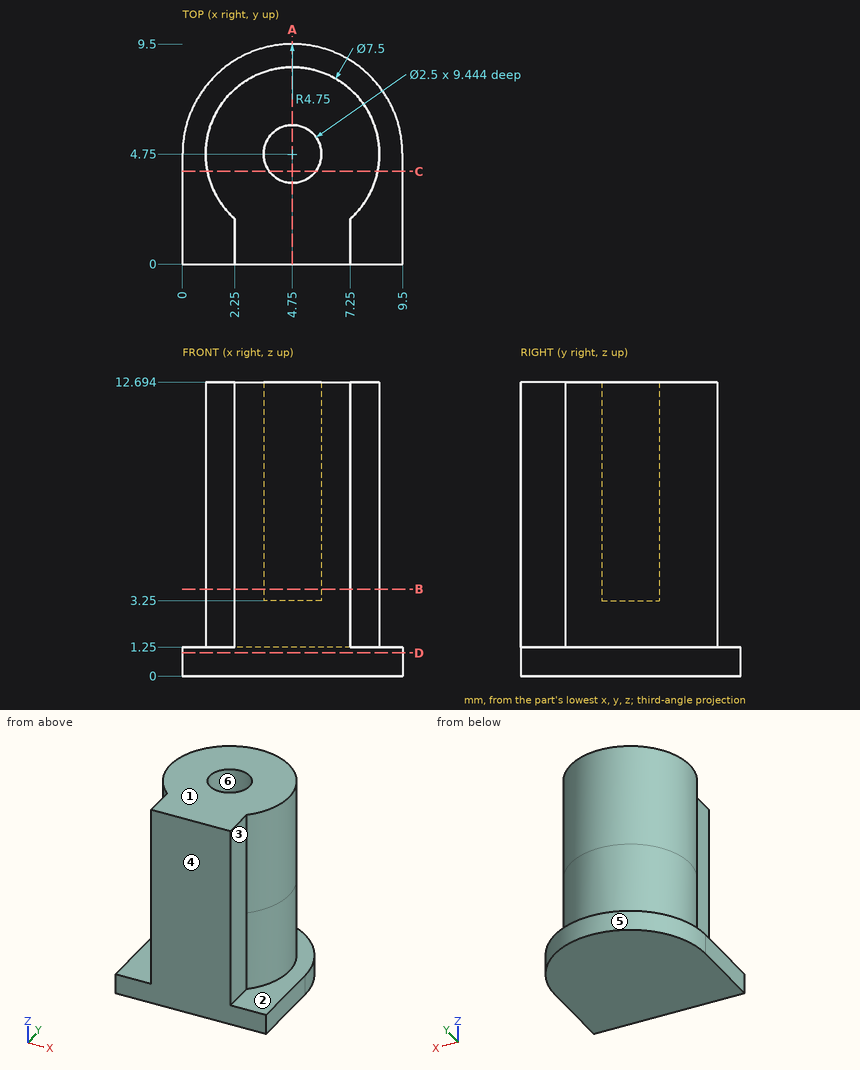
The drawing under review shows one solid part. Ordinate dimensions are in mm from its lowest x, y, z. A direction names the side the tool comes from. Coordinates: 2 decimals unless noted, no trailing zeros. Write each loop counter-clockwise with the first axis right and the second up, starting at its lowest first coordinate (ties: lowest second). Pieces come first, ordered by that corner, then holes. Notation, with made-up numbers: M 32,45.5 L 88,45.5 A33 ccw 88,83.5 Z; hole C 47.5,-6.5 d3. An arc over 180 degrees is marked long. Answer as a JSON object with one key per item and string values.
Item 1: Machinability: for the marked faces 1 and 2, which of the approach directions +Z, -Z, +X, -X, +Y, -Y give a long, thin tool a straight path to every point of the face, cutting with its end or side? Answer none if there is none.
Outcome:
{"face 1": "+Z, +X, -X, +Y, -Y", "face 2": "+Z"}
Item 2: Add section D-D, the plane z = 1. Give the boundary of the cut face in (x, y).
Outcome:
{"outline": "M 0,0 L 9.5,0 L 9.5,4.75 A4.75 ccw 0,4.75 Z"}
Item 3: Draft analysis for pull direction X (two halves, no side actions). For the marked faces 3, 4, 5 and 6, state which applies: pulls with the +X half, pulls with the -X half, needs draft (parallel to the pull), parting line crosses it, or undercut.
Outcome:
{"face 3": "pulls with the +X half", "face 4": "needs draft", "face 5": "parting line crosses it", "face 6": "undercut"}
Item 4: Insertion check: pin 1 Ø5 at (x, z) = (1, 4.5) entering from +Y; pin 2 Ø1 at (y, z) = (7.5, 9) entering from +X; pin 3 Ø5 at (y, z) = (7, 5.5) entering from +X. Each pin has a flat end and moves straight along its axis. Give the tip position at first contact, or say it passes through.
Outcome:
{"pin 1": "y = 8.29", "pin 2": "x = 7.75", "pin 3": "x = 8.5"}
Item 5: Wall thickness on probe 1 along Y at (x, z) = (4.75, 5.5); probe 2 along X at (y, z) = (4.75, 5.5); probe 3 along Z at (x, y) = (8.75, 4.5): over which ranges is each line inside the solid? List them lowest first.
Outcome:
{"probe 1": "0 to 3.5, 6 to 8.5", "probe 2": "1 to 3.5, 6 to 8.5", "probe 3": "0 to 1.25"}
Item 6: Add section C-C, the plane y = 4. Give the boundary of the cut face in (x, z).
Outcome:
{"outline": "M 0,0 L 9.5,0 L 9.5,1.25 L 8.42,1.25 L 8.42,12.69 L 5.75,12.69 L 5.75,3.25 L 3.75,3.25 L 3.75,12.69 L 1.08,12.69 L 1.08,1.25 L 0,1.25 Z"}
Item 7: Add section B-B, the plane z = 3.75. Give the boundary of the cut face in (x, y).
Outcome:
{"outline": "M 2.25,0 L 7.25,0 L 7.25,1.95 A3.75 ccw long 2.25,1.95 Z; hole C 4.75,4.75 d2.5"}
Item 8: Add section A-A, the plane x = 4.75. Give the boundary of the cut face in (y, z), and give its area (3 significant figures).
Outcome:
{"outline": "M 0,0 L 9.5,0 L 9.5,1.25 L 8.5,1.25 L 8.5,12.69 L 6,12.69 L 6,3.25 L 3.5,3.25 L 3.5,12.69 L 0,12.69 Z", "area": "85.5 mm²"}
